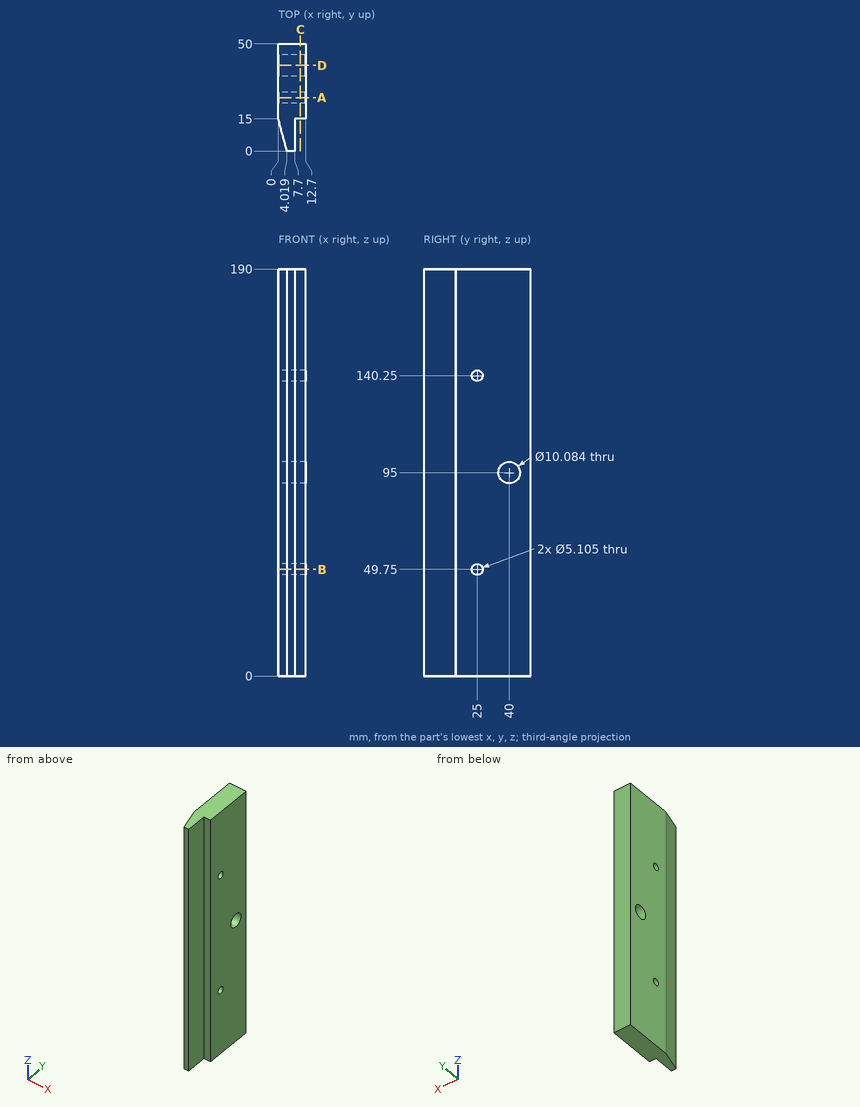
Job drawing, mm, ordinate dimensions from the low corner. One solid piece. Coordinates: 2 decimals unless noted, no trailing zeros. Loops run counter-clockwise (first coordinate to the right, second up) from the corner with the lowest first, then second, coordinate; pieces in that order, holes last. Notation, with made-up numbers: (40.5, 85) - (82.5, 85) arc R30 ccw to (82.5, 107) - close; hole circle Ø5 at (-29, -29). An arc over 180 degrees is marked (long way). Answer as a JSON object with one key per item and string values. Group by question number.
(1) Cut at D-D (y = 40). Give the cut face in (x, z), then the cut area to 4 significant figures.
(2) Cut at A-A (y = 25). Give the cut face in (x, z), then the cut area to 3 significant figures.
(3) Cut at C-C (x = 10.25). State how many separate pieces and enclosed holes the cut face has, then the cut area to 3 significant figures.
(4) Probe line 1 along Y through (x, z) = (5.25, 140.25); line 2 along Y through (x, z) = (9.5, 95); line 3 along Y through (x, z) = (11.75, 101.5). List the from-to ranges inside material, lowest first.
(5) Flat gauge pins, fed straight in: pin 1 (1.5 mm diameter, centred on x = 10.5, z = 91, fed in from -Y); pin 2 (6.5 mm diameter, centred on y = 25, z = 49.75, fed in from -X). Where does each tip first touch, or does it go through?
(6) Cut at B-B (z = 49.75). Give the cut face in (x, y).
Geometry says:
{
 "1": {"outline": "(0, 0) - (12.7, 0) - (12.7, 89.96) - (0, 89.96) - close; (0, 100.04) - (12.7, 100.04) - (12.7, 190) - (0, 190) - close", "area": "2,285 mm^2"},
 "2": {"outline": "(0, 0) - (12.7, 0) - (12.7, 47.2) - (0, 47.2) - close; (0, 52.3) - (12.7, 52.3) - (12.7, 137.7) - (0, 137.7) - close; (0, 142.8) - (12.7, 142.8) - (12.7, 190) - (0, 190) - close", "area": "2,280 mm^2"},
 "3": {"separate pieces": "1", "enclosed holes": "3", "area": "6,530 mm^2"},
 "4": {"line 1": "y = 0 to 22.45, 27.55 to 50", "line 2": "y = 15 to 34.96, 45.04 to 50", "line 3": "y = 15 to 50"},
 "5": {"pin 1": "stops at y = 15", "pin 2": "stops at x = 0"},
 "6": {"outline": "(0, 15) - (4.02, 0) - (7.7, 0) - (7.7, 15) - (12.7, 15) - (12.7, 22.45) - (0, 22.45) - close; (0, 27.55) - (12.7, 27.55) - (12.7, 50) - (0, 50) - close"}
}
